Autodesk Inventor part; units mm, degrees
ref_plane "YZ Plane" through (0, 0, 0) normal (1, 0, 0) x (0, 1, 0)
ref_plane "XZ Plane" through (0, 0, 0) normal (0, 1, 0) x (-1, 0, 0)
ref_plane "XY Plane" through (0, 0, 0) normal (0, 0, 1) x (1, 0, 0)
sketch "Sketch1" plane through (0, 0, 0) normal (1, 0, 0) x (0, 1, 0)
  circle A0 centre (0, 0) radius 20
  line L0 (8.5, 8.5) -> (-16.9, 8.5)
  line L1 (8.5, 8.5) -> (8.5, -16.9)
  line L2 (0, 0) -> (0, 20)
  line L3 (0, 20) -> (-60.9241, 20)
  line L4 (-60.9241, 20) -> (-60.9241, 18.5)
  line L5 (-60.9241, 18.5) -> (0, 18.5)
  line L6 (0, 18.5) -> (0, 20)
  line L7 (0, 0) -> (14.1421, 14.1421)
  line L8 (0, 0) -> (20, 0)
  line L9 (-16.9, 8.5) -> (-16.9, 18.5)
  line L10 (-16.9, 8.5) -> (-22.9, 14.5)
  line L11 (-22.9, 14.5) -> (-22.9, 18.5)
  line L12 (12.3744, 12.3744) -> (12.1502, 13.2109)
  line L13 (11.3137, 13.435) -> (9.2071, 11.3284)
  line L14 (9.4313, 10.4919) -> (10.2678, 10.2678)
  line L15 (8.5, 8.5) -> (8.5, -16.9)
  line L16 (20, 0) -> (20, -60.9241)
  line L17 (20, -60.9241) -> (18.5, -60.9241)
  line L18 (18.5, -60.9241) -> (18.5, 0)
  line L19 (8.5, -16.9) -> (18.5, -16.9)
  line L20 (8.5, -16.9) -> (14.5, -22.9)
  line L21 (14.5, -22.9) -> (18.5, -22.9)
  arc A1 (9.2071, 11.3284) -> (9.4313, 10.4919) centre (9.5607, 10.9749) ccw
  arc A2 (12.1502, 13.2109) -> (11.3137, 13.435) centre (11.6673, 13.0815) ccw
  line L22 (10.4311, 10.4311) -> (9.483, 10.6851)
  arc A3 (9.3485, 11.187) -> (9.483, 10.6851) centre (9.5607, 10.9749) ccw
  line L23 (9.3485, 11.187) -> (11.4551, 13.2936)
  arc A4 (11.957, 13.1591) -> (11.4551, 13.2936) centre (11.6673, 13.0815) ccw
  line L24 (11.957, 13.1591) -> (12.2111, 12.2111)
  point P0 (0, 8.5)
  point P1 (-17.7041, 9.3041)
  point P2 (-16.9, 10.6953)
  dimension "d0" = 40
  dimension "d1" = 25.4
  dimension "d2" = 1.5
  dimension "d4" = 45
  dimension "d6" = 45
  dimension "d7" = 4
  dimension "d8" = 10
  dimension "d10" = 2.5
  dimension "d11" = 2.5
  dimension "d12" = 60
  dimension "d13" = 1.5
  dimension "d15" = 0.5
  dimension "d16" = 0.2
extrude "Extrusion1" add sketch "Sketch1" along normal blind 290 contours L7 L12 A2 L13 A1 L14 L0 L2 A0 | L7 L24 A4 L23 A3 L22 L14 A1 L13 A2 L12 | L5 L2 L0 L9 A0 | A0 L9 L5 | L7 L22 A3 L23 A4 L24 | L9 L10 A0 | A0 L10 L11 L5 L9
sketch "Sketch2" plane through (0, -22.9, 18.5) normal (0, 0, 1) x (1, 0, 0)
  line L0 (0, 22.9) -> (0, 0)
  line L1 (0, 0) -> (290, 0)
  line L2 (290, 22.9) -> (290, 0)
  line L3 (0, 22.9) -> (290, 22.9)
  line L4 (58.3257, 13.1) -> (56.6514, 16)
  line L5 (56.6514, 16) -> (58.3257, 18.9)
  line L6 (58.3257, 18.9) -> (61.6743, 18.9)
  line L7 (61.6743, 18.9) -> (63.3486, 16)
  line L8 (63.3486, 16) -> (61.6743, 13.1)
  line L9 (61.6743, 13.1) -> (58.3257, 13.1)
  line L10 (0, 6) -> (290, 6)
  circle A0 centre (60, 16) radius 1.65
  dimension "d20" = 10
  dimension "d21" = 5.8
  dimension "d22" = 60
  dimension "d25" = 3.3
extrude "Extrusion2" cut sketch "Sketch2" against normal blind 6 contours L4 L5 L6 L7 L8 L9 | A0
extrude "Extrusion3" cut sketch "Sketch2" against normal through all contours A0
sketch "Sketch3" plane through (0, -22.9, 18.5) normal (0, 0, 1) x (1, 0, 0)
  line L0 (0, 37.0421) -> (290, 37.0421)
  line L1 (0, 0) -> (290, 0)
  line L2 (0, 22.9) -> (0, 0)
  line L3 (0, 22.9) -> (0, 37.0421)
  line L4 (2.4384, 37.0421) -> (17.8575, 0)
  line L5 (0, 0) -> (290, 0)
  line L6 (2.4384, 37.0421) -> (0, 42.9)
  point P0 (0, 26.9698)
  dimension "d28" = 112.6
ref_plane "Work Plane1" through (145, 0, 0) normal (-1, 0, 0) x (0, 0, 1)
mirror "Mirror1" about plane through (145, 0, 0) normal (-1, 0, 0) of "Extrusion2", "Extrusion3"
properties part number "ESQUINA_REDONDEADA_R20" material "Steel, Mild, Welded"
Can you work these out from the model? Positions are in its coordinate system, mm. A direction names the side the tool comes from. Give positions to 0.01 mm unless a question says otherwise; leave off trailing zeros. Loops run counter-clockwise (first coordinate to the right, second up) from the corner with the lowest first, then second, coordinate; pieces in that order, holes last. Notation, with made-up numbers: (37.5, 14.25) - (94.5, 14.25) arc R19 cw to (94.5, 44.25) - close; hole circle Ø3 at (68.25, -20.5). An arc over 180 degrees is marked (long way). Return JSON: item names as keys, results as strings.
1. I want a section at A-A on x = 101.5. Please give me the cut outline in (y, z).
Output values:
{"outline": "(-22.9, 14.5) - (-16.9, 8.5) - (8.5, 8.5) - (14.14, 14.14) arc R20 ccw to (0, 20) - (0, 18.5) - (-22.9, 18.5) - close"}
2. I'm going to push flat-ended pins straight in: pin 1 Ø10 at (x, y) = (109, -18) entering from +Z; pin 2 Ø1.7 at (x, y) = (231.5, -7) entering from +Z; pin 3 Ø3 at (x, z) = (187, 18) entering from +Y; pin 4 Ø2.5 at (x, y) = (230, -6.9) entering from -Z. Where does each tip first touch, or does it pass through?
Output values:
{"pin 1": "stops at z = 18.5", "pin 2": "stops at z = 12.5", "pin 3": "stops at y = 11.3", "pin 4": "passes through"}
3. I want a section at C-C on y = 11. Please give me the cut outline in (x, z).
Output values:
{"outline": "(0, 11) - (290, 11) - (290, 16.7) - (0, 16.7) - close"}
4. For faces 4 (the face through (61.4, -5.6, 12.5)), 5 (the face through (143, -12, 18.5)), 6 (the face through (290, -5, 14)), which set-ups out of +Z, -Z, +X, -X, +Y, -Y let a thin tool reach every point of the face, with its end or its side?
Output values:
{"face 4": "+Z", "face 5": "+Z, +X, -X, -Y", "face 6": "+Z, -Z, +X, +Y, -Y"}
5. I want a section at B-B on z = 16.25. Please give me the cut outline in (x, y), and give its area (3 significant figures).
Output values:
{"outline": "(0, -22.9) - (290, -22.9) - (290, 11.66) - (0, 11.66) - close; hole (56.65, -6.9) - (58.33, -9.8) - (61.67, -9.8) - (63.35, -6.9) - (61.67, -4) - (58.33, -4) - close; hole (226.65, -6.9) - (228.33, -9.8) - (231.67, -9.8) - (233.35, -6.9) - (231.67, -4) - (228.33, -4) - close", "area": "9,960 mm²"}
6. We'd pull the mould along Y, two halves only. Please class faces 1 (the face through (143, 7.6, 18.5)), 2 (the face through (231.4, -5.6, 12.5)), 3 (the face through (143, -4, 8.5)): +Y half, -Y half, draft (parallel to the pull), parting line (faces both ways), or undercut.
Output values:
{"face 1": "+Y half", "face 2": "undercut", "face 3": "draft"}
7. If I drill on line 1 (X direction, y = -9.5, z = 13); line 2 (Y direction, x = 60, z = 10.6); line 3 (Y direction, x = 60, z = 11.4), over which ranges is the centre line in solid material (lowest first)?
Output values:
{"line 1": "x = 0 to 58.15, 61.85 to 228.15, 231.85 to 290", "line 2": "y = -19 to -8.55, -5.25 to 10.6", "line 3": "y = -19.8 to -8.55, -5.25 to 11.4"}
